from build123d import *

# Parameters (mm, degrees)
BOSS_EXTRU_1_DEPTH           = 10
ESQUISSE2_R                  = 1.25
ENL_V_MAT_EXTRU_1_DEPTH      = 20
ENL_V_MAT_EXTRU_1_DEPTH_BACK = 10
ENL_V_START                  = 7.5
ESQUISSE2_5_R                = 2.5
ESQUISSE2_5_R_2              = 1.25
ENL_V_MAT_EXTRU_2_DEPTH      = 10
CONG_1_R                     = 1


with BuildPart() as part:
    # Esquisse1 → Boss.-Extru.1 (new body)
    with BuildSketch(Plane.XY):
        with BuildLine():
            Line((3, 20.784609691), (3, 16))
            Line((3, 16), (-3, 16))
            Line((-3, 16), (-3, 20.784609691))
            ThreePointArc((-3, 20.784609691), (-20.993961129, -0.503583277), (-2, -20.90454496))
            Line((-2, -20.90454496), (-2, -15.90454496))
            Line((-2, -15.90454496), (2, -15.90454496))
            Line((2, -15.90454496), (2, -20.90454496))
            ThreePointArc((2, -20.90454496), (20.993961129, -0.503583277), (3, 20.784609691))
        make_face()
        with BuildLine():
            ThreePointArc((9.5, -7.331439149), (0, -12), (-9.5, -7.331439149))
            Line((-9.5, -7.331439149), (-9.5, 7.331439149))
            ThreePointArc((-9.5, 7.331439149), (0, 12), (9.5, 7.331439149))
            Line((9.5, 7.331439149), (9.5, -7.331439149))
        make_face(mode=Mode.SUBTRACT)
    extrude(amount=BOSS_EXTRU_1_DEPTH)

    # Esquisse2 → Enl_v. mat.-Extru.1 (cut, two sides)
    with BuildSketch(Plane(origin=(0, 0, 0), x_dir=(1, 0, 0), z_dir=(0, 1, 0))) as enl_v_mat_extru_1_sk:
        with Locations((15, -5)):
            Circle(ESQUISSE2_R)
        with Locations((-15, -5)):
            Circle(ESQUISSE2_R)
    extrude(amount=ENL_V_MAT_EXTRU_1_DEPTH, mode=Mode.SUBTRACT)
    extrude(enl_v_mat_extru_1_sk.sketch, amount=-ENL_V_MAT_EXTRU_1_DEPTH_BACK, mode=Mode.SUBTRACT)

    # Esquisse2_5 → Enl_v. mat.-Extru.2 (cut)
    with BuildSketch(Plane(origin=(0, 0, 0), x_dir=(1, 0, 0), z_dir=(0, 1, 0)).offset(ENL_V_START)):
        with Locations((15, -5)):
            Circle(ESQUISSE2_5_R)
        with Locations((15, -5)):
            Circle(ESQUISSE2_5_R_2, mode=Mode.SUBTRACT)
        with Locations((-15, -5)):
            Circle(ESQUISSE2_5_R)
        with Locations((-15, -5)):
            Circle(ESQUISSE2_5_R_2)
    extrude(amount=ENL_V_MAT_EXTRU_2_DEPTH, mode=Mode.SUBTRACT)

    # Cong_1
    cong_1_edges = [part.edges().sort_by_distance(p)[0] for p in [
        (-2, -18.40454496, 0),
        (-2, -18.40454496, 10),
        (0, -15.90454496, 0),
        (0, -15.90454496, 10),
        (2, -18.40454496, 0),
        (2, -18.40454496, 10),
        (-20.993961129, -0.503583277, 0),
        (-20.993961129, -0.503583277, 10),
        (-3, 18.392304845, 0),
        (-3, 18.392304845, 10),
        (0, 16, 0),
        (0, 16, 10),
        (3, 18.392304845, 0),
        (3, 18.392304845, 10),
        (20.993961129, -0.503583277, 0),
        (20.993961129, -0.503583277, 10),
    ]]
    fillet(cong_1_edges, radius=CONG_1_R)


solid = part.part
Source: CAD feature listing. Evaluate the final solid. Frame: model axes, mm. A direction names the side the tool comes from. Round coordinates to 2 decimals unless told otherwise and drop trailing zeros. Loops run counter-clockwise (first coordinate to the right, second up) from the corner with the lowest first, then second, coordinate; pieces in that order, holes last. Notation, with made-up numbers: (84, -14) -> (109, -14) arc R7 ccw to (109, -4) -> close; hole circle Ø9 at (-23, -20). An arc over 180 degrees is marked (long way). Answer as a JSON object with one key per item and string values. Group by question number.
Q1. Section query D-D (z = 5). Output: boundary loops of the cut face in (x, y), plus the area to 3 significant figures.
Q2. Ray query, line 1 (Z direction, x = -15, y = 9.75); line 2 (Z direction, x = 15, y = -3.5); line 3 (X direction, y = -2.5, z = 5). Return the intervals inside material, ascending. Write a range as from..to.
Q3. Section query A-A (z = 1.5). Output: boundary loops of the cut face in (x, y), plus the area to 3 significant figures.
Q4. Mould query, pull axis Z, two halves, no side actions, for faces 1 (the cylindrical face through (2.301, -17.947, 9.715)), 2 (the cylindrical face through (0.042, -15.604, 0.285)), 3 (the flat face through (14, 7.5, 6)). Classes: pulls with the +Z half, pulls with the -Z half, needs draft (parallel to the pull), parting line crosses it, or undercut.
Q5. Contact query for flat-ended pins moving along their axis: P1, Ø2.5, axis at y = 17.5, z = 7, coming from the -X side; P2, Ø2, axis at x = -9.5, y = -5.5, coming from the -Z side; P3, Ø3, axis at x = -15.5, z = 4.5, coming from the +Y side; P4, Ø2, axis at x = -0.5, z = 5.5, coming from the -Y side. Output: stop coordinate, or through.
Q6. Section query B-B (x = 1.5). Output: boundary loops of the cut face in (y, z).
Q7. Section query C-C (y = 9). State how many separate pieces and enclosed holes the cut face has, plus the area to 3 significant figures.
Q8. Access query for faces 4 (the cylindrical face through (0, -12, 5)), 5 (the flat face through (15, -10, 5)), 6 (the flat face through (3, 18, 5)), 7 (the cylindrical face through (-3.301, 17.933, 0.285)). Directions: +Z, -Z, +X, -X, +Y, -Y. A direction counts if a zero-diameter tool reaches every point of the face in a straight line with its end or side. Return the directions, or none.
Completed:
{
 "1": {"outline": "(-17.5, 7.5) -> (-17.5, 11.61) arc R21 ccw to (-2, -20.9) -> (-2, -15.9) -> (2, -15.9) -> (2, -20.9) arc R21 ccw to (17.5, 11.61) -> (17.5, 7.5) -> (16.25, 7.5) -> (16.25, -10) -> (13.75, -10) -> (13.75, 7.5) -> (12.5, 7.5) -> (12.5, 16.87) arc R21 ccw to (3, 20.78) -> (3, 16) -> (-3, 16) -> (-3, 20.78) arc R21 ccw to (-12.5, 16.87) -> (-12.5, 7.5) -> (-13.75, 7.5) -> (-13.75, -10) -> (-16.25, -10) -> (-16.25, 7.5) -> close; hole (-9.5, -7.33) arc R12 ccw to (9.5, -7.33) -> (9.5, 7.33) arc R12 ccw to (-9.5, 7.33) -> close", "area": "775 mm²"},
 "2": {"line 1": "0..2.5, 7.5..10", "line 2": "0..3.75, 6.25..10", "line 3": "-20.85..-16.25, -13.75..-9.5, 9.5..13.75, 16.25..20.85"},
 "3": {"outline": "(-3, 16) -> (-3, 20.78) arc R21 ccw to (-2, -20.9) -> (-2, -15.9) -> (2, -15.9) -> (2, -20.9) arc R21 ccw to (3, 20.78) -> (3, 16) -> close; hole (-9.5, -7.33) arc R12 ccw to (9.5, -7.33) -> (9.5, 7.33) arc R12 ccw to (-9.5, 7.33) -> close", "area": "933 mm²"},
 "4": {"face 1": "pulls with the +Z half", "face 2": "pulls with the -Z half", "face 3": "undercut"},
 "5": {"P1": "x = -13.3", "P2": "z = 0", "P3": "y = 7.5", "P4": "y = -15.9"},
 "6": {"outline": "(-15.9, 1) arc R1 ccw to (-14.9, 0) -> (-11.91, 0) -> (-11.91, 10) -> (-14.9, 10) arc R1 ccw to (-15.9, 9) -> close; (11.91, 0) -> (15, 0) arc R1 ccw to (16, 1) -> (16, 9) arc R1 ccw to (15, 10) -> (11.91, 10) -> close"},
 "7": {"separate pieces": "2", "enclosed holes": "2", "area": "181 mm²"},
 "8": {"face 4": "+Z, -Z", "face 5": "+Y", "face 6": "+Z, -Z, +Y", "face 7": "-Z, +Y"}
}
